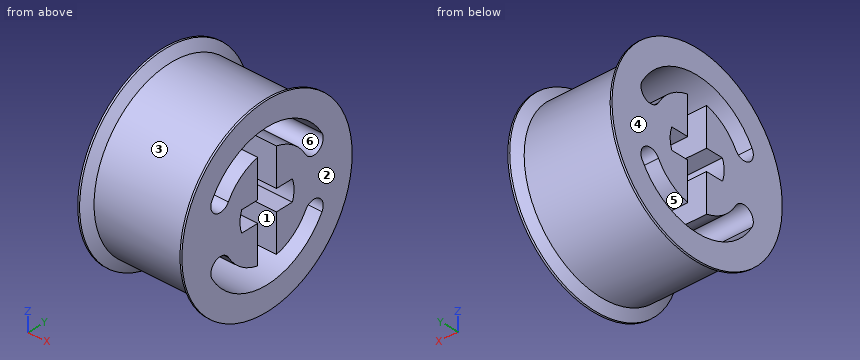
Autodesk Inventor part; units mm, degrees
ref_plane "YZ Plane" through (0, 0, 0) normal (1, 0, 0) x (0, 1, 0)
ref_plane "XZ Plane" through (0, 0, 0) normal (0, 1, 0) x (-1, 0, 0)
ref_plane "XY Plane" through (0, 0, 0) normal (0, 0, 1) x (1, 0, 0)
sketch "Sketch1" plane through (0, 0, 0) normal (0, 0, 1) x (1, 0, 0)
  line L0 (0, -1.5) -> (0, 9) construction
  line L1 (-4, 7.25) -> (-3.8557, 7.25)
  line L2 (-3.8557, 7.25) -> (-3.4226, 6.5)
  line L3 (-3.4226, 6.5) -> (3.4226, 6.5)
  line L4 (3.4226, 6.5) -> (3.8557, 7.25)
  line L5 (3.8557, 7.25) -> (4, 7.25)
  line L6 (4, 7.25) -> (4, 0)
  line L7 (4, 0) -> (-4, 0)
  line L8 (-4, 0) -> (-4, 7.25)
  point P0 (0, 0)
  point P1 (0, 6.5)
  point P2 (4, 7.5)
  dimension "d0" = 13
  dimension "d1" = 60
  dimension "d2" = 8
  dimension "d3" = 15
  dimension "d4" = 14.5
revolve "Revolution1" add sketch "Sketch1" angle 360 about axis through (4, 0, 0) along (-1, 0, 0)
sketch "Sketch2" plane through (0, 0, 0) normal (1, 0, 0) x (0, 1, 0)
  circle A0 centre (0, 0) radius 2.3
  line L0 (0.8, 2.1564) -> (0.8, 0.8)
  line L1 (0.8, -0.8) -> (0.8, -2.1564)
  line L2 (-2.1564, 0.8) -> (-0.8, 0.8)
  line L3 (0.8, 0.8) -> (2.1564, 0.8)
  line L4 (2.1564, -0.8) -> (0.8, -0.8)
  line L5 (-0.8, -0.8) -> (-2.1564, -0.8)
  line L6 (-0.8, 2.1564) -> (-0.8, 0.8)
  line L7 (-0.8, -0.8) -> (-0.8, -2.1564)
  dimension "d6" = 4.6
  dimension "d7" = 1.6
extrude "Extrusion1" cut sketch "Sketch2" along normal through all both and the other way through all contours A0 L4 L1 L7 L5 L2 L6 L0 L3
sketch "Sketch3" plane through (0, 0, 0) normal (1, 0, 0) x (0, 1, 0)
  circle A0 centre (0, 0) radius 2.3 construction
  arc A1 (3.2909, 1.9) -> (-3.2909, 1.9) centre (0, 0) ccw
  arc A2 (4.6765, 2.7) -> (-4.6765, 2.7) centre (0, 0) ccw
  arc A3 (-3.2909, -1.9) -> (3.2909, -1.9) centre (0, 0) ccw
  arc A4 (-4.6765, -2.7) -> (4.6765, -2.7) centre (0, 0) ccw
  arc A5 (3.2909, 1.9) -> (4.6765, 2.7) centre (3.9837, 2.3) ccw
  arc A6 (4.6765, -2.7) -> (3.2909, -1.9) centre (3.9837, -2.3) ccw
  arc A7 (-4.6765, 2.7) -> (-3.2909, 1.9) centre (-3.9837, 2.3) ccw
  arc A8 (-3.2909, -1.9) -> (-4.6765, -2.7) centre (-3.9837, -2.3) ccw
  line L0 (-3.9837, 2.3) -> (0, 0) construction
  line L1 (0, 0) -> (3.9837, 2.3) construction
  line L2 (3.9837, -2.3) -> (0, 0) construction
  line L3 (-3.9837, -2.3) -> (0, 0) construction
  line L4 (0, -6.16) -> (0, 6.16) construction
  line L5 (-5.8947, 0) -> (5.8947, 0) construction
  dimension "d10" = 1.6
  dimension "d11" = 120
  dimension "d12" = 120
  dimension "d15" = 3.8
extrude "Extrusion2" cut sketch "Sketch3" along normal through all both and the other way through all
sketch "Sketch4" plane through (0, 0, 0) normal (1, 0, 0) x (0, 1, 0)
  arc A0 (3.2909, 1.9) -> (-3.2909, 1.9) centre (0, 0) ccw
  arc A1 (-3.2909, -1.9) -> (3.2909, -1.9) centre (0, 0) ccw
  line L0 (0.8, -0.8) -> (0.8, -2.1564) construction
  line L1 (-0.8, -2.1564) -> (-0.8, -0.8) construction
  line L2 (0.8, 3.7148) -> (0.8, -3.7148)
  line L3 (-0.8, 3.7148) -> (-0.8, -3.7148)
extrude "Extrusion3" cut sketch "Sketch4" along normal through all both and the other way through all
properties part number "LEGO Brick 3482" material "Steel"
Geometry check sheet. Reference: the model listing, model coordinates, mm. Face numbers are marked on the shaded views. A direction names the side the tool comes from. Give positions to 0.01 mm unless a question says otherwise; leave off trailing zeros. Loops run counter-clockwise (first coordinate to the right, second up) from the corner with the lowest first, then second, coordinate; pieces in that order, holes last.
(1) Section check A-A on y = 0. Record the cut outline in (x, z).
From the geometry:
outline: (-4, -7.25) - (-3.86, -7.25) - (-3.42, -6.5) - (3.42, -6.5) - (3.86, -7.25) - (4, -7.25) - (4, -5.4) - (-4, -5.4) - close; (-4, 5.4) - (4, 5.4) - (4, 7.25) - (3.86, 7.25) - (3.42, 6.5) - (-3.42, 6.5) - (-3.86, 7.25) - (-4, 7.25) - close
(2) Depth check by flat-ended pin: pin 1 Ø3 at (x, z) = (-0.5, 4.5) entering from +Y; pin 2 Ø1.5 at (x, z) = (-1, 2.5) entering from -Y; pin 3 Ø1.5 at (x, z) = (0.5, -2) entering from +Y; pin 4 Ø8 at (y, z) = (0, 1) entering from -X. Enter the tip coordinate at first touch or a pass-through.
From the geometry:
pin 1: stops at y = 5.77
pin 2: stops at y = -6.26
pin 3: stops at y = 6.38
pin 4: stops at x = -4
(3) Section check C-C on x = -1. Record the cut outline in (y, z).
From the geometry:
outline: circle Ø13 at (0, 0); hole (-4.68, -2.7) arc R5.4 ccw to (4.68, -2.7) arc R0.8 ccw to (3.29, -1.9) arc R3.8 cw to (0.8, -3.71) - (0.8, -0.8) - (2.16, -0.8) arc R2.3 ccw to (2.16, 0.8) - (0.8, 0.8) - (0.8, 3.71) arc R3.8 cw to (3.29, 1.9) arc R0.8 ccw to (4.68, 2.7) arc R5.4 ccw to (-4.68, 2.7) arc R0.8 ccw to (-3.29, 1.9) arc R3.8 cw to (-0.8, 3.71) - (-0.8, 0.8) - (-2.16, 0.8) arc R2.3 ccw to (-2.16, -0.8) - (-0.8, -0.8) - (-0.8, -3.71) arc R3.8 cw to (-3.29, -1.9) arc R0.8 ccw to start
(4) Thickness scan on L1, parallel to Y at x = -2.5, z = -2.75; L2, parallel to Z at x = -2.75, y = 3.5; L3, parallel to Z at x = -1, y = -2. Record the ranges inside material, lowest first.
From the geometry:
L1: y = -5.89 to -4.65, -2.62 to -0.8, 0.8 to 2.62, 4.65 to 5.89
L2: z = -5.48 to -4.11, -1.66 to 1.66, 4.11 to 5.48
L3: z = -6.18 to -5.02, -3.23 to -0.8, 0.8 to 3.23, 5.02 to 6.18
(5) Release check for a two-part mould opening along Z. For the marked faces 3, 4, 5 and 6 record: released by +Z, released by -Z, zero draft, split by the parting line, or undercut.
From the geometry:
face 3: split by the parting line
face 4: zero draft
face 5: undercut
face 6: undercut
(6) Set-up check for the marked faces 1 and 2: record each of +Z, -Z, +X, -X, +Y, -Y from which the full face is reachable in a straight line by a thin tool's end or side.
From the geometry:
face 1: +X, -X
face 2: +Z, -Z, +X, +Y, -Y
(7) Section check D-D on z = -2.3. Count the separate pieces of the cut face and the enclosed holes in it, then the cut area to 3 significant figures.
From the geometry:
separate pieces: 4
enclosed holes: 0
area: 57.5 mm2
(8) Section check B-B on z = 0. Record the cut outline in (x, y), then the cut area to 3 significant figures.
From the geometry:
outline: (-4, -7.25) - (-3.86, -7.25) - (-3.42, -6.5) - (3.42, -6.5) - (3.86, -7.25) - (4, -7.25) - (4, -2.3) - (-4, -2.3) - close; (-4, 2.3) - (4, 2.3) - (4, 7.25) - (3.86, 7.25) - (3.42, 6.5) - (-3.42, 6.5) - (-3.86, 7.25) - (-4, 7.25) - close
area: 68.3 mm2
